Work out the finished part from the listing and answer in its coordinate system (mm). A direction names the side the tool comes from. Give positions to 0.01 mm unless a question says otherwise; leave off trailing zeros. Order: outer loops, then holes, each group sorted by start corner. A loop starts at its lowest first (then second) coordinate and runs counter-clockwise, first axis right, second up. Notation, with made-up numbers: (-18, 71) -> (40, 71) arc R19 cw to (40, 76) -> close; hole circle Ø7 at (-39.75, 46.25). An arc over 180 degrees is marked (long way). Use a Markdown table: item, result. Add a question column.
```python
from build123d import *
from OCP.BRepAlgoAPI import BRepAlgoAPI_Cut
from OCP.TopTools import TopTools_ListOfShape

# Parameters (mm, degrees)
BOSS_EXTRUDE1_DEPTH    = 60
CUT_EXTRUDE1_START     = -130
CUT_EXTRUDE1_OUTLINE_R = 4
CUT_EXTRUDE1_OUTLINE_W = 2.5
CUT_EXTRUDE1_OUTLINE_H = 5.5
CUT_EXTRUDE1_DEPTH     = 130
CUT_EXTRUDE2_REACH     = 93.924
SKETCH3_R              = 11
SKETCH3_R_2            = 1.5
SKETCH3_R_3            = 5
SKETCH3_R_4            = 2.5
SKETCH4_R              = 1.5
CUT_EXTRUDE3_DEPTH     = 94.407708115


with BuildPart() as part:
    # Sketch1 → Boss-Extrude1 (new body)
    with BuildSketch(Plane(origin=(0, 0, 0), x_dir=(0, 0, -1), z_dir=(1, 0, 0))):
        Polygon((-65, 0), (65, 0), (65, 30), (60, 30), (60, 5), (-60, 5), (-60, 30), (-65, 30), align=None)
    extrude(amount=BOSS_EXTRUDE1_DEPTH)


with BuildPart() as cut_extrude1_tool:
    # Cut-Extrude1: read off the stored shape, not the designer's step
    # Cut-Extrude1 outline → Cut-Extrude1 (new body)
    with BuildSketch(Plane(origin=(0, 0, -65), x_dir=(-1, 0, 0), z_dir=(0, 0, -1)).offset(CUT_EXTRUDE1_START)):
        with BuildLine():
            Line((0, 30), (-30, 29.999998923))
            ThreePointArc((-30, 29.999998923), (-27.525092827, 29.688901535), (-25.204173103, 28.774965689))
            Line((-25.204173103, 28.774965689), (-3.642920811, 16.99098415))
            ThreePointArc((-3.642920811, 16.99098415), (-0.979221216, 14.419252925), (0, 10.848507507))
            Line((0, 10.848507507), (0, 30))
        make_face()
        with BuildLine():
            ThreePointArc((-60, 10.848507507), (-59.020778784, 14.419252925), (-56.357079189, 16.99098415))
            Line((-56.357079189, 16.99098415), (-34.795826897, 28.774965689))
            ThreePointArc((-34.795826897, 28.774965689), (-32.474907173, 29.688901535), (-30, 29.999998923))
            Line((-30, 29.999998923), (-60, 30))
            Line((-60, 30), (-60, 10.848507507))
        make_face()
        with Locations((-30, 20)):
            Circle(CUT_EXTRUDE1_OUTLINE_R)
        with Locations((-20, 20)):
            Rectangle(CUT_EXTRUDE1_OUTLINE_W, CUT_EXTRUDE1_OUTLINE_H)
        with Locations((-40, 20)):
            Rectangle(CUT_EXTRUDE1_OUTLINE_W, CUT_EXTRUDE1_OUTLINE_H)
    extrude(amount=CUT_EXTRUDE1_DEPTH)


with BuildPart() as part_1:
    add(part.part)

    # Cut-Extrude1: cut by cut_extrude1_tool, with a tolerance
    cut_extrude1_stock = TopTools_ListOfShape()
    cut_extrude1_stock.Append(part_1.part.wrapped)
    cut_extrude1_tools = TopTools_ListOfShape()
    cut_extrude1_tools.Append(cut_extrude1_tool.part.wrapped)
    cut_extrude1_cut = BRepAlgoAPI_Cut()
    cut_extrude1_cut.SetArguments(cut_extrude1_stock)
    cut_extrude1_cut.SetTools(cut_extrude1_tools)
    cut_extrude1_cut.SetFuzzyValue(0.00001)
    cut_extrude1_cut.Build()
    add(Compound.cast(cut_extrude1_cut.Shape()).solids(), mode=Mode.REPLACE)

    # Sketch3 → Cut-Extrude2 (cut, up to next)
    with BuildSketch(Plane(origin=(0, 5, 0), x_dir=(1, 0, 0), z_dir=(0, 1, 0)), mode=Mode.PRIVATE) as cut_extrude2_sk1:
        with Locations(Location((30, 35, 0), (0, 0, 270))):
            Circle(SKETCH3_R)
    cut_extrude2_tool1 = extrude(cut_extrude2_sk1.sketch, amount=-CUT_EXTRUDE2_REACH, mode=Mode.PRIVATE) & part_1.part
    # Sketch3 → Cut-Extrude2 (cut, up to next)
    with BuildSketch(Plane(origin=(0, 5, 0), x_dir=(1, 0, 0), z_dir=(0, 1, 0)), mode=Mode.PRIVATE) as cut_extrude2_sk2:
        with Locations(Location((45.5, 19.5, 0), (0, 0, 270))):
            Circle(SKETCH3_R_2)
    cut_extrude2_tool2 = extrude(cut_extrude2_sk2.sketch, amount=-CUT_EXTRUDE2_REACH, mode=Mode.PRIVATE) & part_1.part
    # Sketch3 → Cut-Extrude2 (cut, up to next)
    with BuildSketch(Plane(origin=(0, 5, 0), x_dir=(1, 0, 0), z_dir=(0, 1, 0)), mode=Mode.PRIVATE) as cut_extrude2_sk3:
        with Locations(Location((45.5, 50.5, 0), (0, 0, 270))):
            Circle(SKETCH3_R_2)
    cut_extrude2_tool3 = extrude(cut_extrude2_sk3.sketch, amount=-CUT_EXTRUDE2_REACH, mode=Mode.PRIVATE) & part_1.part
    # Sketch3 → Cut-Extrude2 (cut, up to next)
    with BuildSketch(Plane(origin=(0, 5, 0), x_dir=(1, 0, 0), z_dir=(0, 1, 0)), mode=Mode.PRIVATE) as cut_extrude2_sk4:
        with Locations(Location((14.5, 50.5, 0), (0, 0, 270))):
            Circle(SKETCH3_R_2)
    cut_extrude2_tool4 = extrude(cut_extrude2_sk4.sketch, amount=-CUT_EXTRUDE2_REACH, mode=Mode.PRIVATE) & part_1.part
    # Sketch3 → Cut-Extrude2 (cut, up to next)
    with BuildSketch(Plane(origin=(0, 5, 0), x_dir=(1, 0, 0), z_dir=(0, 1, 0)), mode=Mode.PRIVATE) as cut_extrude2_sk5:
        with Locations(Location((14.5, 19.5, 0), (0, 0, 270))):
            Circle(SKETCH3_R_2)
    cut_extrude2_tool5 = extrude(cut_extrude2_sk5.sketch, amount=-CUT_EXTRUDE2_REACH, mode=Mode.PRIVATE) & part_1.part
    # Sketch3 → Cut-Extrude2 (cut, up to next)
    with BuildSketch(Plane(origin=(0, 5, 0), x_dir=(1, 0, 0), z_dir=(0, 1, 0)), mode=Mode.PRIVATE) as cut_extrude2_sk6:
        with Locations(Location((30, -30, 0), (0, 0, 270))):
            Circle(SKETCH3_R_3)
    cut_extrude2_tool6 = extrude(cut_extrude2_sk6.sketch, amount=-CUT_EXTRUDE2_REACH, mode=Mode.PRIVATE) & part_1.part
    # Sketch3 → Cut-Extrude2 (cut, up to next)
    with BuildSketch(Plane(origin=(0, 5, 0), x_dir=(1, 0, 0), z_dir=(0, 1, 0)), mode=Mode.PRIVATE) as cut_extrude2_sk7:
        with Locations(Location((48.25, -30, 0), (0, 0, 270))):
            Circle(SKETCH3_R_4)
    cut_extrude2_tool7 = extrude(cut_extrude2_sk7.sketch, amount=-CUT_EXTRUDE2_REACH, mode=Mode.PRIVATE) & part_1.part
    # Sketch3 → Cut-Extrude2 (cut, up to next)
    with BuildSketch(Plane(origin=(0, 5, 0), x_dir=(1, 0, 0), z_dir=(0, 1, 0)), mode=Mode.PRIVATE) as cut_extrude2_sk8:
        with Locations(Location((11.75, -30, 0), (0, 0, 270))):
            Circle(SKETCH3_R_4)
    cut_extrude2_tool8 = extrude(cut_extrude2_sk8.sketch, amount=-CUT_EXTRUDE2_REACH, mode=Mode.PRIVATE) & part_1.part
    add(cut_extrude2_tool1.solids().sort_by_distance((30, 5, -35))[0], mode=Mode.SUBTRACT)
    add(cut_extrude2_tool2.solids().sort_by_distance((45.5, 5, -19.5))[0], mode=Mode.SUBTRACT)
    add(cut_extrude2_tool3.solids().sort_by_distance((45.5, 5, -50.5))[0], mode=Mode.SUBTRACT)
    add(cut_extrude2_tool4.solids().sort_by_distance((14.5, 5, -50.5))[0], mode=Mode.SUBTRACT)
    add(cut_extrude2_tool5.solids().sort_by_distance((14.5, 5, -19.5))[0], mode=Mode.SUBTRACT)
    add(cut_extrude2_tool6.solids().sort_by_distance((30, 5, 30))[0], mode=Mode.SUBTRACT)
    add(cut_extrude2_tool7.solids().sort_by_distance((48.25, 5, 30))[0], mode=Mode.SUBTRACT)
    add(cut_extrude2_tool8.solids().sort_by_distance((11.75, 5, 30))[0], mode=Mode.SUBTRACT)

    # Sketch4 → Cut-Extrude3 (cut, through all)
    with BuildSketch(Plane.ZY):
        with Locations((62.5, 20)):
            Circle(SKETCH4_R)
        with Locations((-62.5, 20)):
            Circle(SKETCH4_R)
    extrude(amount=-CUT_EXTRUDE3_DEPTH, mode=Mode.SUBTRACT)


solid = part_1.part
```
1) Determine the mould class of faces 1 (the flat face through (41.25, 19, 61)), 2 (the cylindrical face through (9.3, 2.5, 29.5)), 3 (the flat face through (30, 12, 65)) for opening direction Z: released by +Z, released by -Z, zero draft, split by the parting line, or undercut.
2) Which of the six approach directions +Z, -Z, +X, -X, +Y, -Y give full straight-line access (tool end or side, diameter ignored) to faces 4 (the cylindrical face through (59.05, 14.37, -62.46)), 5 (the flat face through (20, 17.25, -62))?
3) The part is cut by section D-D, the plane x = 55. Determine the outline of the cut face in (y, z).
4) Flat-ended cylindrical pins translate along their axes: pin 1 (1.2 mm diameter, centred on x = 39.5, z = 62.5, fed in from +Y); pin 2 (6 mm diameter, centred on x = 48.25, z = 30, fed in from +Y); pin 3 (5.5 mm diameter, centred on y = 21, z = 62.5, fed in from +X). Find the tip coordinate at first contact, or state that the pin passes through.
5) The part is cut by section C-C, the plane z = -32. Determine the outline of the cut face in (x, y).
6) The part is cut by section B-B, the plane y = 12.5. Determine the outline of the cut face in (x, z), then the cut area to 3 significant figures.
7) The part is cut by section A-A, the plane z = -50.5. Determine the outline of the cut face in (x, y).
8) Straight lines are drawn through the part: line 1 (X direction, y = 1.65, z = 30); line 2 (Z direction, x = 37, y = 9); line 3 (X direction, y = 2.4, z = -35). For each, find the intervals that lie inside material, in ascending order.
A:
| question | item | result |
|---|---|---|
| 1 | face 1 | zero draft |
| 1 | face 2 | undercut |
| 1 | face 3 | released by +Z |
| 2 | face 4 | +Z, -Z, +X, +Y |
| 2 | face 5 | +Z, -Z |
| 3 | outline | (0, -65) -> (17.73, -65) -> (17.73, -60) -> (5, -60) -> (5, 60) -> (17.73, 60) -> (17.73, 65) -> (0, 65) -> close |
| 4 | pin 1 | y = 26.53 |
| 4 | pin 2 | y = 5 |
| 4 | pin 3 | x = 54.05 |
| 5 | outline | (0, 0) -> (19.42, 0) -> (19.42, 5) -> (0, 5) -> close; (40.58, 0) -> (60, 0) -> (60, 5) -> (40.58, 5) -> close |
| 6 | outline | (0.2, -65) -> (59.8, -65) -> (59.8, -60) -> (0.2, -60) -> close; (0.2, 60) -> (59.8, 60) -> (59.8, 65) -> (0.2, 65) -> close |
| 6 | area | 596 mm^2 |
| 7 | outline | (0, 0) -> (13, 0) -> (13, 5) -> (0, 5) -> close; (16, 0) -> (44, 0) -> (44, 5) -> (16, 5) -> close; (47, 0) -> (60, 0) -> (60, 5) -> (47, 5) -> close |
| 8 | line 1 | 0 to 9.25, 14.25 to 25, 35 to 45.75, 50.75 to 60 |
| 8 | line 2 | -65 to -60, 60 to 65 |
| 8 | line 3 | 0 to 19, 41 to 60 |
